Geometry: final body of the model. Coordinates: model frame, mm. A direction names the side the tool comes from. Give positions to 0.01 mm unless a question says otherwise; leave off trailing zeros. Write each loop counter-clockwise with the first axis right and the second up, starting at its lowest first coordinate (ties: lowest second). Pieces come first, ordered by that corner, then holes.
Q1. Draft query along Z for faces 4 (the face through (-11, 7, 50)), 5 (the face through (0, 7, 43.8)), 6 (the face through (19, 7, 50)), 7 (the face through (14.3, 8, 50)). Return one class per face: pulls with the +Z half, pulls with the -Z half, needs draft (parallel to the pull), parting line crosses it, or undercut.
Q2. Cut plane D-D on y = 0. Return the cut outline in (x, z).
Q3. Line query: L1, parallel to Y at x = -21.5, z = 48.3; L2, parallel to Z at x = 18, y = 7; L3, parallel to Y at x = 16, z = 51.25. Output: solid intervals per line, ascending.
Q4. Cut plane B-B on y = -26.5. Return the cut outline in (x, z), plus the area to 3 significant figures.
Q5. Cut plane C-C on z = 56. Return the cut outline in (x, y), plus the area to 3 significant figures.
Q6. Cut plane A-A on x = -18. Return the cut outline in (y, z).
Q7. Pin query (flat end, axial travel): pin 1 (4 mm diameter, centred on x = 5.5, z = 52, fed in from +Y); pin 2 (3 mm diameter, centred on x = 15, z = 50, fed in from +Y); pin 3 (3 mm diameter, centred on x = 2.5, z = 47, fed in from +Y). Return the tip coordinate at first contact, or that it passes through.
Q8. Reachability of faces 1 (the face through (15.63, 8.47, 45.65)), 2 (the face through (0.02, 15.56, 46.56)), 3 (the face through (0, -1.5, 46.6)) from +Z, -Z, +X, -X, +Y, -Y: full face, straight path, thin tool, end or side. Return the list, or none.
```python
from build123d import *

# Parameters (mm, degrees)
PAD007_DEPTH               = 2.7
CYLINDER1015_R             = 1.7
CYLINDER1015_DEPTH         = 100
CLONE008_PITCH_ANGLE       = 90
PAD006_DEPTH               = 82
PAD009_DEPTH               = 40
CHAMFER011_SIZE            = 1
CHAMFER011_PLACEMENT_ANGLE = 180


with BuildPart() as clone_of_m3nuthousingmaster:
    # Sketch008 → Pad007 (new body)
    with BuildSketch(Plane(origin=(65, 30, 1.5), x_dir=(0, 0, 1), z_dir=(-1, 0, 0))):
        Polygon((0, 0), (1.674316, 2.9), (21.674316, 2.9), (21.674316, -2.9), (1.674316, -2.9), align=None)
    extrude(amount=PAD007_DEPTH)


with BuildPart() as clone_of_m3nuthousingmaster_1:
    # Clone009 placement: moved
    add(clone_of_m3nuthousingmaster.part.moved(Location((-117, -0.99996, 1.5))))


with BuildPart() as fusion021:
    # Cylinder1015 → Cylinder1015 (new body)
    with BuildSketch(Plane.XY):
        Circle(CYLINDER1015_R)
    extrude(amount=CYLINDER1015_DEPTH)


with BuildPart() as fusion021_1:
    # Clone008 pitch: moved
    add(fusion021.part.rotate(Axis((0, 0, 0), (0, 1, 0)), CLONE008_PITCH_ANGLE))


with BuildPart() as fusion021_2:
    # Clone008 placement: moved
    add(fusion021_1.part.moved(Location((-58, 29, 6.5))))

    # Fusion021: union Clone of M3NutHousingMaster
    add(clone_of_m3nuthousingmaster_1.part)


with BuildPart() as pad006:
    # Sketch007 → Pad006 (new body)
    with BuildSketch(Plane(origin=(0, 0, 0), x_dir=(-1, 0, 0), z_dir=(0, 1, 0))):
        Polygon((0, 0), (0, 20), (5, 20), (5, 10), (18, 10), (18, 0), align=None)
    extrude(amount=PAD006_DEPTH)


with BuildPart() as clone_of_lateraladjust:
    # Sketch010 → Pad009 (new body)
    with BuildSketch(Plane(origin=(-18, 29, 2), x_dir=(0, 1, 0), z_dir=(1, 0, 0))):
        Polygon((-12.5, 0), (-5.35926, 5), (-5.35926, 8), (5.35926, 8), (5.35926, 5), (12.5, 0), align=None)
    extrude(amount=-PAD009_DEPTH)

    # Fusion034: union Pad006
    add(pad006.part)

    # Cut025: cut Fusion021
    add(fusion021_2.part, mode=Mode.SUBTRACT)

    # Chamfer011
    chamfer011_edges = [clone_of_lateraladjust.edges().sort_by_distance(p)[0] for p in [
        (-38, 16.5, 2),
        (-38, 41.5, 2),
    ]]
    chamfer(chamfer011_edges, length=CHAMFER011_SIZE)


with BuildPart() as clone_of_lateraladjust_1:
    # Chamfer011 placement: moved
    add(clone_of_lateraladjust.part.moved(Location((-37.7, 79, 44))).rotate(Axis((-37.7, 79, 44), (0, 0, 1)), CHAMFER011_PLACEMENT_ANGLE))


with BuildPart() as clone_of_lateraladjust_2:
    # Clone088 placement: moved
    add(clone_of_lateraladjust_1.part.moved(Location((0, -43, -2.2))))


solid = clone_of_lateraladjust_2.part
```
Data:
1. face 4: undercut
1. face 5: pulls with the -Z half
1. face 6: undercut
1. face 7: needs draft
2. outline: (-37.7, 41.8) - (-19.7, 41.8) - (-19.7, 43.8) - (20.3, 43.8) - (20.3, 47.65) - (-19.7, 47.65) - (-19.7, 51.8) - (-32.7, 51.8) - (-32.7, 61.8) - (-37.7, 61.8) - close
3. L1: y = -46 to 5.3, 8.7 to 36
3. L2: z = 43.8 to 46.6, 50 to 51.8
3. L3: y = 1.64 to 4.1, 9.9 to 12.36
4. outline: (-37.7, 41.8) - (-19.7, 41.8) - (-19.7, 51.8) - (-32.7, 51.8) - (-32.7, 61.8) - (-37.7, 61.8) - close
4. area: 230 mm2
5. outline: (-37.7, -46) - (-32.7, -46) - (-32.7, 36) - (-37.7, 36) - close
5. area: 410 mm2
6. outline: (-4.68, 44.37) - (-4.5, 43.8) - (18.5, 43.8) - (18.68, 44.37) - (12.36, 48.8) - (12.36, 51.8) - (1.64, 51.8) - (1.64, 48.8) - close; hole circle Ø3.4 at (7, 48.3)
7. pin 1: stops at y = 12.36
7. pin 2: stops at y = 12.79
7. pin 3: stops at y = 17.07
8. face 1: +Z
8. face 2: +Z, +X, +Y
8. face 3: +Z, +X, -Y
